Autodesk Inventor part; units mm, degrees
ref_plane "作業平面1" through (0, 0.5, 0) normal (0, -1, 0) x (1, 0, 0)
ref_plane "YZ Plane" through (0, 0, 0) normal (1, 0, 0) x (0, 1, 0)
ref_plane "XZ Plane" through (0, 0, 0) normal (0, 1, 0) x (-1, 0, 0)
sketch "スケッチ1" plane through (0, 0, 0) normal (0, 1, 0) x (-1, 0, 0)
  circle A0 centre (0, 0) radius 3
  dimension "d0" = 6
extrude "押し出し1" add sketch "スケッチ1" along normal blind 12
sketch "スケッチ4" plane through (0, 12, 0) normal (0, 1, 0) x (1, 0, 0)
  circle A0 centre (0, 0) radius 1
  dimension "d7" = 2
extrude "押し出し4" add sketch "スケッチ4" along normal blind 0.5
fillet "フィレット1" radius 0.2 2 edges at (-1, 12, 0) (3, 12, 0)
ref_plane "作業平面1" through (0, 0.5, 0) normal (0, -1, 0) x (1, 0, 0)
split_face "分割1"
sketch "スケッチ6" plane through (0, 12.5, 0) normal (0, 1, 0) x (1, 0, 0)
  circle A0 centre (0, 0) radius 0.4
  dimension "d12" = 0.8
extrude "押し出し5" add sketch "スケッチ6" along normal blind 3.5
properties part number "CoreLessMotor"
Design review of the part built by this model. Coordinates are the model's own, in mm. A direction names the side the tool comes from. Give positions to 0.01 mm unless a question says otherwise; leave off trailing zeros. Loops run counter-clockwise (first coordinate to the right, second up) from the corner with the lowest first, then second, coordinate; pieces in that order, holes last. Notation, with made-up numbers: M 53,52 L 75,52 A17 cw 75,83 Z; hole C 2,0 d9. An arc over 180 degrees is marked long. One line per question, with ' | ' between items. Start each with the question number.
1. Add section D-D (y = 8). Write out the cut boundary in (x, z), plus the area to 3 significant figures.
2. Add section B-B (x = 0). Write out the cut boundary in (y, z), plus the area to 3 significant figures.
3. For faces 1 (the face through (0.46, 12.35, -0.89)), 2 (the face through (3, 6, 0)), list the 3-axis set-ups (+Z, -Z, +X, -X, +Y, -Y) from which the entire face can be reached by the end or side of a thin tool; tool diameter is ignored.
4. To check wall thickness, follow L1, parallel to X at y = 4, z = 2.75; L2, parallel to Y at x = 1, z = -2.5. State the ranges of each line that lie inside material, in increasing order.
5. Add section A-A (z = 0). Write out the cut boundary in (x, y), plus the area to 3 significant figures.
6. Insertion check: P1, Ø3, axis at x = 0, z = -0.5, coming from the +Y side; P2, Ø1, axis at x = -2, y = 10.5, coming from the -Z side; P3, Ø2, axis at x = 1.5, z = 0.5, coming from the +Y side. Each pin has a flat end and moves straight along its axis. Give the tip position at first contact, or say it passes through.
7. Add section C-C (y = 13.75). Write out the cut boundary in (x, z).
Worked out:
1) outline: C 0,0 d6 | area: 28.3 mm²
2) outline: M 0,-3 L 11.8,-3 A0.2 ccw 12,-2.8 L 12,-1.2 A0.2 cw 12.2,-1 L 12.5,-1 L 12.5,-0.4 L 16,-0.4 L 16,0.4 L 12.5,0.4 L 12.5,1 L 12.2,1 A0.2 cw 12,1.2 L 12,2.8 A0.2 ccw 11.8,3 L 0,3 Z | area: 75.8 mm²
3) face 1: +Y | face 2: +Y, -Y
4) L1: x = -1.2 to 1.2 | L2: y = 0 to 12
5) outline: M -3,0 L 3,0 L 3,11.8 A0.2 ccw 2.8,12 L 1.2,12 A0.2 cw 1,12.2 L 1,12.5 L 0.4,12.5 L 0.4,16 L -0.4,16 L -0.4,12.5 L -1,12.5 L -1,12.2 A0.2 cw -1.2,12 L -2.8,12 A0.2 ccw -3,11.8 Z | area: 75.8 mm²
6) P1: stops at y = 16 | P2: stops at z = -2.6 | P3: stops at y = 12.5
7) outline: C 0,0 d0.8
